from build123d import *

# Parameters (mm, degrees)
BOSS_EXTRUDE1_DEPTH       = 7
M6X1_0_TAPPED_HOLE1_D     = 5
M6X1_0_TAPPED_HOLE1_DEPTH = 15
M6X1_0_TAPPED_HOLE1_TIP   = 1.502151548
SKETCH5_R                 = 3.175
CUT_EXTRUDE1_DEPTH        = 1.5


with BuildPart() as part:
    # Sketch1 → Boss-Extrude1 (new body)
    with BuildSketch(Plane.XY):
        Polygon((0, 5.773502692), (-5, 2.886751346), (-5, -2.886751346), (0, -5.773502692), (5, -2.886751346), (5, 2.886751346), align=None)
    extrude(amount=BOSS_EXTRUDE1_DEPTH)

    # M6x1.0 Tapped Hole1
    with Locations(Plane.XY.offset(7)):
        with Locations((0, 0)):
            Hole(M6X1_0_TAPPED_HOLE1_D / 2, depth=M6X1_0_TAPPED_HOLE1_DEPTH)
            with Locations((0, 0, -(M6X1_0_TAPPED_HOLE1_DEPTH + M6X1_0_TAPPED_HOLE1_TIP / 2))):  # 118° drill point
                Cone(0, M6X1_0_TAPPED_HOLE1_D / 2, M6X1_0_TAPPED_HOLE1_TIP, mode=Mode.SUBTRACT)

    # Sketch4 → Cut-Revolve1 (revolve, cut)
    with BuildSketch(Plane(origin=(0, 0, 0), x_dir=(0, 0, -1), z_dir=(1, 0, 0)), mode=Mode.PRIVATE) as cut_revolve1_sk:
        Polygon((-6.553418013, 5.773502692), (-7, 5), (-7, 5.773502692), align=None)
        Polygon((0, 5.773502692), (-0.446581987, 5.773502692), (0, 5), align=None)
    revolve(cut_revolve1_sk.sketch.rotate(Axis((0, 0, 0), (0, 0, 1)), 270), axis=Axis((0, 0, 0), (0, 0, 1)), mode=Mode.SUBTRACT)

    # Sketch5 → Cut-Extrude1 (cut)
    with BuildSketch(Plane.XY.offset(7)):
        Circle(SKETCH5_R)
    extrude(amount=-CUT_EXTRUDE1_DEPTH, mode=Mode.SUBTRACT)


solid = part.part
Can you work these out from the model? Positions are in its coordinate system, mm. Round coordinates to 2 decimals unless told otherwise and drop trailing zeros. Loops run counter-clockwise (first coordinate to the right, second up) from the corner with the lowest first, then second, coordinate; pieces in that order, holes last. Notation, with made-up numbers: (55.5, -24) - (81.5, -24) arc R31 cw to (81.5, 10) - close; hole circle Ø11 at (68.25, 40). An arc over 180 degrees is marked (long way). Write item = value, one per line. Start each with the question number.
(1) For P1, Ø1, axis at x = 3, z = 3, coming from the +Y side; P2, Ø1, axis at y = -3.5, z = 5, coming from the +X side; P3, Ø2, axis at x = 0.5, z = 5.5, coming from the +Y side, each with a flat end and sliding along its axis, tell me the tip position at first contact or that it passes through.
(2) If we section it at A-A (z = 1): Please give me the cut outline in (x, y), and give its area (3 significant figures).
(3) If I drill on probe 1 along Y at (x, z) = (0.5, 6.75); probe 2 along Y at (x, z) = (0.5, 1.75); probe 3 along Z at (x, y) = (1.25, 2.5), over which ranges is the centre line in solid material (lowest first)? Write a range as [from, to].
(4) If we mould it in two halves opening along X, with no side actions, what happens to faces 1 (the face through (0.013, 5.184, 6.894)), 2 (the face through (-0.69, -3.1, 6.26)), 3 (the face through (2, -2, 0))? For each: released by +X, released by -X, zero draft, split by the parting line, or undercut.
Ans:
q1.P1 = 4.33
q1.P2 = 4.8
q1.P3 = 5.77
q2.outline = (-5, -2.89) - (0, -5.77) - (5, -2.89) - (5, 2.89) - (0, 5.77) - (-5, 2.89) - close; hole circle Ø5 at (0, 0)
q2.area = 67.0 mm²
q3.probe_1 = [-5.41, -3.14], [3.14, 5.41]
q3.probe_2 = [-5.48, -2.45], [2.45, 5.48]
q3.probe_3 = [0, 5.5]
q4.face_1 = split by the parting line
q4.face_2 = undercut
q4.face_3 = zero draft
